CAD build for the part. Positions are in the model's coordinates, mm. A direction names the side the tool comes from. Round coordinates to 2 decimals unless told otherwise and drop trailing zeros. Write each loop counter-clockwise with the first axis right and the second up, starting at its lowest first coordinate (ties: lowest second). Pieces come first, ordered by that corner, then holes. Notation, with made-up numbers: (-37, 57) -> (-30, 57) arc R22 cw to (-30, 64) -> close; hole circle Ø9 at (-5, -26.75). An arc over 180 degrees is marked (long way). Put each result on its own line as item: value. Start each with the question number.
1. 3-axis set-ups, long thin cutter, end or side, ignore diameter. For faces 1 (the flat face through (-17, -25.4, -1)), 2 (the flat face through (-9.525, 27, -1)), 3 (the flat face through (27, -2.921, -1)): which of +Z, -Z, +X, -X, +Y, -Y reach the whole face in a straight line?
2. Saw through at C-C on y = 0. List the corners of the cut face in (x, z) (3 decimals), and give its area (3 significant figures).
3. Drill centre lines: line 1 (X direction, y = 25.5, z = -2.75) (3 decimals); line 2 (Y direction, x = 0, z = -2.1) (3 decimals); line 3 (X direction, y = 0, z = -2.25) (3 decimals). Where is each one in solid material? Low to high. Write a range as from..to.
4. Saw through at A-A on x = 0. List the corners of the cut face in (y, z) (3 decimals), and give its area (3 significant figures).
5. Flat gauge pins, fed straight in: P1, Ø1.5, axis at y = -13, z = -2, coming from the +X side; P2, Ø0.9, axis at x = -2.5, z = -1, coming from the +Y side; P3, Ø0.9, axis at x = -27, z = -1.5, coming from the -Y side. Where does each tip first touch, or does it go through?
6. Saw through at B-B on z = -1.15. List the corners of the cut face in (x, y) (3 decimals), and give its area (3 significant figures).
7. Saw through at D-D on x = 12. List the corners of the cut face in (y, z).
8. Pull direction X, two halves, no side cores. Call faces 4 (the flat face through (27, 16.129, -1)), 5 (the flat face through (0, 25.4, -1)), 6 (the flat face through (-9.525, -27, -1)): pulls with the +X half, pulls with the -X half, needs draft (parallel to the pull), parting line crosses it, or undercut.
Autodesk Inventor part; units mm, degrees
ref_plane "YZ Plane" through (0, 0, 0) normal (1, 0, 0) x (0, 1, 0)
ref_plane "XZ Plane" through (0, 0, 0) normal (0, 1, 0) x (-1, 0, 0)
ref_plane "XY Plane" through (0, 0, 0) normal (0, 0, 1) x (1, 0, 0)
sketch "Sketch1" plane through (0, 0, 0) normal (0, 0, 1) x (1, 0, 0)
  line L0 (-28.321, -28.321) -> (28.321, -28.321)
  line L1 (28.321, -28.321) -> (28.321, 28.321)
  line L2 (28.321, 28.321) -> (-28.321, 28.321)
  line L3 (-28.321, 28.321) -> (-28.321, -28.321)
  line L4 (-28.321, -28.321) -> (28.321, 28.321) construction
  line L5 (28.321, -28.321) -> (-28.321, 28.321) construction
  point P0 (0, 0)
  dimension "d0" = 56.642
  dimension "d1" = 56.642
extrude "Extrusion1" add sketch "Sketch1" against normal blind 2.921
sketch "Sketch4" plane through (0, 0, 0) normal (0, 0, 1) x (1, 0, 0)
  line L0 (-28.321, -28.321) -> (-9.525, -28.321)
  line L1 (-9.525, -28.321) -> (-9.525, -25.4)
  line L2 (-9.525, -25.4) -> (-28.321, -25.4)
  line L3 (-28.321, -25.4) -> (-28.321, -28.321)
  line L4 (28.321, 28.321) -> (-28.321, 28.321)
  line L5 (-28.321, 28.321) -> (-28.321, -28.321)
  line L6 (-9.525, 28.321) -> (9.525, 28.321)
  line L7 (9.525, 28.321) -> (9.525, 25.4)
  line L8 (9.525, 25.4) -> (-9.525, 25.4)
  line L9 (-9.525, 25.4) -> (-9.525, 28.321)
  line L10 (-28.321, -28.321) -> (-25.4, -28.321)
  line L11 (-25.4, -28.321) -> (-25.4, -2.921)
  line L12 (-25.4, -2.921) -> (-28.321, -2.921)
  line L13 (-28.321, -2.921) -> (-28.321, -28.321)
  line L14 (-28.321, 28.321) -> (-25.4, 28.321)
  line L15 (-25.4, 28.321) -> (-25.4, 16.129)
  line L16 (-25.4, 16.129) -> (-28.321, 16.129)
  line L17 (-28.321, 16.129) -> (-28.321, 28.321)
  line L18 (0, -3.175) -> (0, -6.3407)
  line L19 (28.321, -28.321) -> (9.525, -28.321)
  line L20 (9.525, -28.321) -> (9.525, -25.4)
  line L21 (9.525, -25.4) -> (28.321, -25.4)
  line L22 (28.321, -25.4) -> (28.321, -28.321)
  line L23 (28.321, 28.321) -> (28.321, -28.321)
  line L24 (9.525, 25.4) -> (9.525, 28.321)
  line L25 (28.321, -28.321) -> (25.4, -28.321)
  line L26 (25.4, -28.321) -> (25.4, -2.921)
  line L27 (25.4, -2.921) -> (28.321, -2.921)
  line L28 (28.321, -2.921) -> (28.321, -28.321)
  line L29 (28.321, 28.321) -> (25.4, 28.321)
  line L30 (25.4, 28.321) -> (25.4, 16.129)
  line L31 (25.4, 16.129) -> (28.321, 16.129)
  line L32 (28.321, 16.129) -> (28.321, 28.321)
  line L33 (-28.321, -28.321) -> (28.321, -28.321)
  point P0 (0, 0)
  point P1 (28.321, 0.1976)
  dimension "d16" = 2.921
  dimension "d37" = 9.525
  dimension "d38" = 18.796
  dimension "d44" = 2.921
  dimension "d45" = 19.05
  dimension "d46" = 18.796
  dimension "d53" = 25.4
  dimension "d54" = 19.05
  dimension "d55" = 2.921
  dimension "d56" = 2.921
  dimension "d57" = 12.192
  dimension "d58" = 18.796
  dimension "d59" = 19.05
  dimension "d60" = 12.192
  dimension "d61" = 19.05
  dimension "d62" = 25.4
extrude "Extrusion5" cut sketch "Sketch4" against normal blind 25.4 contours L3 L2 L11 L0 | L11 L2 L1 L0 | L5 L12 L11 L2 | L20 L21 L26 L19 | L5 L4 L15 L16 | L26 L21 L22 L19 | L26 L27 L23 L21 | L4 L7 L8 L9 | L31 L30 L4 L23
hole "Hole1" at (0, 0, 0) direction (0, 0, -1) diameter 19.05 end through all
equation "\"d1\" = d0"
equation "\"d38\" = -d37 + 0.5 * d0"
equation "\"d44\" = d16"
equation "\"d45\" = d42"
equation "\"d46\" = d38"
equation "\"d55\" = d16"
equation "\"d56\" = d16"
equation "\"d59\" = d45"
equation "\"d19\" = 0.5 * d0"
equation "\"d48\" = 0.5 * d0"
equation "\"d42\" = 2 * d37"
properties part number "SideB"
Return value:
1. face 1: +Z, -Z, -X, -Y
1. face 2: +Z, -Z, +Y
1. face 3: +Z, -Z, +X, -Y
2. outline: (-28.321, -2.921) -> (-9.525, -2.921) -> (-9.525, 0) -> (-28.321, 0) -> close; (9.525, -2.921) -> (28.321, -2.921) -> (28.321, 0) -> (9.525, 0) -> close
2. area: 110 mm^2
3. line 1: x = -25.4..-9.525, 9.525..25.4
3. line 2: y = -28.321..-9.525, 9.525..25.4
3. line 3: x = -28.321..-9.525, 9.525..28.321
4. outline: (-28.321, -2.921) -> (-9.525, -2.921) -> (-9.525, 0) -> (-28.321, 0) -> close; (9.525, -2.921) -> (25.4, -2.921) -> (25.4, 0) -> (9.525, 0) -> close
4. area: 101 mm^2
5. P1: stops at x = 25.4
5. P2: stops at y = 25.4
5. P3: stops at y = -2.92
6. outline: (-28.321, -2.921) -> (-25.4, -2.921) -> (-25.4, -25.4) -> (-9.525, -25.4) -> (-9.525, -28.321) -> (9.525, -28.321) -> (9.525, -25.4) -> (25.4, -25.4) -> (25.4, -2.921) -> (28.321, -2.921) -> (28.321, 16.129) -> (25.4, 16.129) -> (25.4, 28.321) -> (9.525, 28.321) -> (9.525, 25.4) -> (-9.525, 25.4) -> (-9.525, 28.321) -> (-25.4, 28.321) -> (-25.4, 16.129) -> (-28.321, 16.129) -> close; hole circle Ø19.05 at (0, 0)
6. area: 2,560 mm^2
7. outline: (-25.4, -2.92) -> (28.32, -2.92) -> (28.32, 0) -> (-25.4, 0) -> close
8. face 4: needs draft
8. face 5: undercut
8. face 6: pulls with the -X half
